Geometry: final body of the model. Coordinates: model frame, mm. Face numbers are marked on the shaded views. Round coordinates to 2 decimals unless told otherwise and drop trailing zeros. Loops run counter-clockwise (first coordinate to the right, second up) from the corner with the lowest first, then second, coordinate; pieces in that order, holes last. Notation, with made-up numbers: M -24.75,85 L 13.25,85 A27 cw 13.25,124 Z; hole C -6.5,73.5 d11. An arc over 180 degrees is marked long. Answer as a JSON object with one key per item and string values.
Autodesk Inventor part; units mm, degrees
ref_plane "YZ Plane" through (0, 0, 0) normal (1, 0, 0) x (0, 1, 0)
ref_plane "XZ Plane" through (0, 0, 0) normal (0, 1, 0) x (-1, 0, 0)
ref_plane "XY Plane" through (0, 0, 0) normal (0, 0, 1) x (1, 0, 0)
sketch "Esquisse1" plane through (0, 0, 0) normal (0, 0, 1) x (1, 0, 0)
  arc A0 (22.8757, 107.3508) -> (1.1243, 107.3508) centre (12, 109) ccw
  arc A1 (9.0085, 2.7745) -> (14.9915, 2.7745) centre (12, 3) ccw
  line L0 (1, 109) -> (9.0085, 2.7745)
  line L1 (23, 109) -> (14.9915, 2.7745)
  point P0 (0, 0)
  dimension "d2" = 22
extrude "Extrusion1" add sketch "Esquisse1" along normal blind 5 contours L1 A1 L0 A0
sketch "Esquisse2" plane through (23, 109, 5) normal (0.9971701, -0.075178, 0) x (0, 0, -1)
  line L0 (5, -109.527) -> (0, -109.527)
  line L1 (2.5, -109.527) -> (1.5, -109.527)
  line L2 (2.5, -109.527) -> (3.5, -109.527)
  line L3 (3.5, -109.527) -> (3.5, -104.527)
  line L4 (3.5, -104.527) -> (1.5, -104.527)
  line L5 (1.5, -104.527) -> (1.5, -109.527)
  point P0 (5, -110.4206)
  dimension "d6" = 1
  dimension "d7" = 1
  dimension "d8" = 5
  dimension "d9" = 2
extrude "Extrusion2" cut sketch "Esquisse2" against normal through all
sketch "Esquisse3" plane through (0, 0, 0) normal (0, 0, -1) x (-1, 0, 0)
  arc A0 (-14.9915, 2.7745) -> (-9.0085, 2.7745) centre (-12, 3) ccw
  arc A1 (-1, 109) -> (-23, 109) centre (-12, 109) ccw
  circle A2 centre (-12, 109) radius 4
  arc A3 (-14.9915, 2.7745) -> (-9.0085, 2.7745) centre (-12, 3) ccw
  line L0 (-12, 0) -> (-12, 2)
  circle A4 centre (-12, 2) radius 1
  line L1 (-14.8284, 2) -> (-9.1716, 2)
  point P0 (0, 0)
  dimension "d13" = 8
  dimension "d24" = 2
  dimension "d25" = 2
  dimension "d26" = 5.6569
extrude "Extrusion3" cut sketch "Esquisse3" against normal through all contours L1 L0 A4 | A4 L1 | L0 L1 A4 | A2
sketch "Esquisse8" plane through (0, 0, 5) normal (0, 0, 1) x (1, 0, 0)
  circle A0 centre (12, 109) radius 4
  line L0 (12, 109) -> (12, 65.6)
  line L1 (12, 65.6) -> (12, 67.6)
  line L2 (12, 67.6) -> (14, 67.6)
  line L3 (14, 67.6) -> (14, 63.6)
  line L4 (14, 63.6) -> (10, 63.6)
  line L5 (10, 63.6) -> (10, 67.6)
  line L6 (10, 67.6) -> (12, 67.6)
  point P0 (0, 0)
  dimension "d27" = 43.4
  dimension "d29" = 2
  dimension "d30" = 2
  dimension "d31" = 4
  dimension "d32" = 4
extrude "Extrusion5" add sketch "Esquisse8" along normal blind 12 contours L2 L3 L4 L5 L6
properties part number "Jambe"
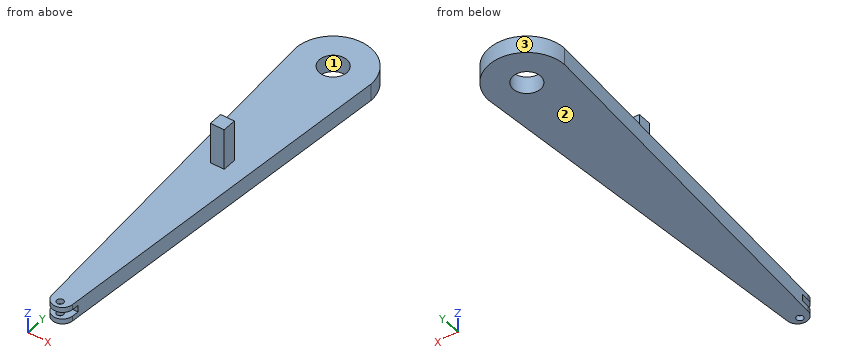
1) Section query B-B (z = 15.25). Return the cut outline in (x, y), and give its area (3 significant figures).
Results:
{"outline": "M 10,63.6 L 14,63.6 L 14,67.6 L 10,67.6 Z", "area": "16.0 mm2"}
2) Ray query, line 1 (Y direction, x = 12, z = 0.55); line 2 (Z direction, x = 6, y = 94); line 3 (X direction, y = 97.5, z = 2.25). Return the intervals inside material, ascending.
Results:
{"line 1": "0 to 1, 3 to 105, 113 to 120", "line 2": "0 to 5", "line 3": "1.87 to 22.13"}
3) Section query A-A (x = 12). Return the cut outline in (y, z), and give its area (3 significant figures).
Results:
{"outline": "M 0,0 L 1,0 L 1,1.5 L 0,1.5 Z; M 0,3.5 L 1,3.5 L 1,5 L 0,5 Z; M 3,0 L 105,0 L 105,5 L 67.6,5 L 67.6,17 L 63.6,17 L 63.6,5 L 3,5 L 3,3.5 L 5.01,3.5 L 5.01,1.5 L 3,1.5 Z; M 113,0 L 120,0 L 120,5 L 113,5 Z", "area": "592 mm2"}
4) Pin query (flat end, axial travel): P1, Ø2.5, axis at x = 11, y = 1.5, coming from the +Z side; P2, Ø1.2, axis at x = 12, y = 2, coming from the +Z side; P3, Ø3, axis at y = 65.5, z = 9, coming from the +X side; P4, Ø4.5, axis at x = 11.5, z = 10.5, coming from the +Y side. Return the tip coordinate at first contact, or that it passes through.
Results:
{"P1": "z = 5", "P2": "through", "P3": "x = 14", "P4": "y = 67.6"}
5) Section query C-C (y = 43). Return the cut outline in (x, z).
Results:
{"outline": "M 5.98,0 L 18.02,0 L 18.02,5 L 5.98,5 Z"}
6) Pull-direction query (X, two-part tool) for the marked faces 1, 2 and 3; classes: +X half, -X half, draft (parallel to the pull), parting line (faces both ways), or undercut.
Results:
{"face 1": "undercut", "face 2": "draft", "face 3": "parting line"}
